```python
from build123d import *

# Parameters (mm, degrees)
F0_W     = 55.88
F0_H     = 105.1052
F0_R     = 1.7145
F0_W_2   = 48.26
F0_H_2   = 10.4902
F1_DEPTH = 3.175
F2_R     = 1.016
F3_DEPTH = 105.1062
F4_R     = 1.7145
F4_W     = 9.3726
F4_H     = 6.35
F4_W_2   = 6.223
F4_H_2   = 10.414
F4_W_3   = 8.3566
F4_H_3   = 15.24
F5_DEPTH = 3.175
F6_W     = 7.62
F6_H     = 10.16
F6_W_2   = 5.08
F6_H_2   = 6.35
F7_DEPTH = 25.4
F8_R     = 1.6002
F9_R     = 3.175
F10_F1_R = 1.016
F10_F2_R = 1.016


# Not quite as in the source:
# - a feature names something its author has since deleted; it is built from what else it names


with BuildPart() as f1:
    # F0 (on Top) → F1 (new body)
    with BuildSketch(Plane.XY):
        Rectangle(F0_W, F0_H)
        with Locations((-17.9451, -29.5656)):
            Circle(F0_R, mode=Mode.SUBTRACT)
        with Locations((-9.8679, -47.7901)):
            Circle(F0_R, mode=Mode.SUBTRACT)
        with Locations((9.8679, -47.7901)):
            Circle(F0_R, mode=Mode.SUBTRACT)
        with Locations((-9.8679, 15.0622)):
            Circle(F0_R, mode=Mode.SUBTRACT)
        with Locations((0, 37.7825)):
            Rectangle(F0_W_2, F0_H_2, mode=Mode.SUBTRACT)
        with Locations((-9.8679, 47.7901)):
            Circle(F0_R, mode=Mode.SUBTRACT)
        with Locations((9.8679, 15.0622)):
            Circle(F0_R, mode=Mode.SUBTRACT)
        with Locations((9.8679, 47.7901)):
            Circle(F0_R, mode=Mode.SUBTRACT)
    extrude(amount=F1_DEPTH)

    # F2 (on face) → F3 (cut, through all)
    with BuildSketch(Plane.XZ.offset(52.5526)):
        Circle(F2_R)
    extrude(amount=-F3_DEPTH, mode=Mode.SUBTRACT)

    # F4 (on face) → F5 (join)
    with BuildSketch(Plane.XY.offset(3.175)):
        Polygon((-7.3914, 17.7927), (-20.5994, 17.7927), (-20.5994, 14.8093839596), (-20.5994, 9.8679), (-14.7574, 9.8679), (-14.7574, 13.9827), (-11.8364, 13.9827), (-11.8364, 12.2047), (-7.3914, 12.2047), (-7.3914, 13.9827), align=None)
        with Locations((-9.8679, 15.0622)):
            Circle(F4_R, mode=Mode.SUBTRACT)
        with Locations((11.3157, 14.6177)):
            Rectangle(F4_W, F4_H)
        with Locations((9.8679, 15.0622)):
            Circle(F4_R, mode=Mode.SUBTRACT)
        with Locations((-17.4879, -28.6893)):
            Rectangle(F4_W_2, F4_H_2)
        with Locations((-17.9451, -29.5656)):
            Circle(F4_R, mode=Mode.SUBTRACT)
        with Locations((16.2687, -22.6695)):
            Rectangle(F4_W_3, F4_H_3)
    extrude(amount=F5_DEPTH)

    # F6 (on face) → F7 (cut)
    with BuildSketch(Plane(origin=(0, 0, 0), x_dir=(1, 0, 0), z_dir=(0, 0, -1))):
        with Locations((14.9225, 4.4323)):
            Rectangle(F6_W, F6_H)
        with Locations((-13.6525, 2.5273)):
            Rectangle(F6_W_2, F6_H_2)
    extrude(amount=-F7_DEPTH, mode=Mode.SUBTRACT)

    # F8
    f8_edges = [f1.edges().sort_by_distance(p)[0] for p in [
        (-16.1925, 0.6477, 1.5875),
        (11.1125, 0.6477, 1.5875),
        (18.7325, 0.6477, 1.5875),
        (18.7325, -9.5123, 1.5875),
        (11.1125, -9.5123, 1.5875),
        (-16.1925, -5.7023, 1.5875),
        (-11.1125, -5.7023, 1.5875),
        (-11.1125, 0.6477, 1.5875),
    ]]
    fillet(f8_edges, radius=F8_R)

    # F9
    f9_edges = [f1.edges().sort_by_distance(p)[0] for p in [
        (-24.13, 32.5374, 1.5875),
        (24.13, 32.5374, 1.5875),
        (24.13, 43.0276, 1.5875),
        (-24.13, 43.0276, 1.5875),
    ]]
    fillet(f9_edges, radius=F9_R)

    # F10: fillet of radius 1.016 on 34 edges, made by hand

    # F10_f1
    f10_f1_edges = [f1.edges().sort_by_distance(p)[0] for p in [
        (-7.3914, 17.7927, 4.7625),
        (6.6294, 17.7927, 4.7625),
        (16.002, 17.7927, 4.7625),
        (20.447, -15.0495, 4.7625),
        (12.0904, -15.0495, 4.7625),
        (20.447, -30.2895, 4.7625),
        (12.0904, -30.2895, 4.7625),
        (-14.3764, -33.8963, 4.7625),
        (-20.5994, -33.8963, 4.7625),
        (-14.3764, -23.4823, 4.7625),
        (-20.5994, -23.4823, 4.7625),
        (6.6294, 11.4427, 4.7625),
        (16.002, 11.4427, 4.7625),
        (-20.5994, 17.7927, 4.7625),
        (-20.5994, 9.8679, 4.7625),
        (-14.7574, 9.8679, 4.7625),
        (-7.3914, 12.2047, 4.7625),
        (-11.8364, 12.2047, 4.7625),
    ]]
    fillet(f10_f1_edges, radius=F10_F1_R)

    # F10_f2
    f10_f2_edges = [f1.edges().sort_by_distance(p)[0] for p in [
        (-14.3764, -28.6893, 3.175),
        (20.447, -22.6695, 3.175),
        (16.002, 14.6177, 3.175),
        (-7.3914, 14.9987, 3.175),
        (-20.5994, -28.6893, 3.175),
        (-17.4879, -23.4823, 3.175),
        (-17.4879, -33.8963, 3.175),
        (16.2687, -30.2895, 3.175),
        (16.2687, -15.0495, 3.175),
        (12.0904, -22.6695, 3.175),
        (-13.9954, 17.7927, 3.175),
        (-20.5994, 13.8303, 3.175),
        (-17.6784, 9.8679, 3.175),
        (11.3157, 11.4427, 3.175),
        (11.3157, 17.7927, 3.175),
        (6.6294, 14.6177, 3.175),
        (6.9269795103, 17.4951204897, 3.175),
        (6.9269795103, 11.7402795103, 3.175),
        (15.7044204897, 17.4951204897, 3.175),
        (15.7044204897, 11.7402795103, 3.175),
        (-20.3018204897, 10.1654795103, 3.175),
        (-15.0549795103, 10.1654795103, 3.175),
        (-20.3018204897, 17.4951204897, 3.175),
        (-7.6889795103, 17.4951204897, 3.175),
        (12.3879795103, -15.3470795103, 3.175),
        (12.3879795103, -29.9919204897, 3.175),
        (20.1494204897, -15.3470795103, 3.175),
        (20.1494204897, -29.9919204897, 3.175),
        (-20.3018204897, -33.5987204897, 3.175),
        (-14.6739795103, -33.5987204897, 3.175),
        (-14.6739795103, -23.7798795103, 3.175),
        (-20.3018204897, -23.7798795103, 3.175),
        (-7.6889795103, 12.5022795103, 3.175),
    ]]
    fillet(f10_f2_edges, radius=F10_F2_R)


solid = f1.part
```
Can you work these out from the model? Positions are in its coordinate system, mm. A direction names the side the tool comes from. Round coordinates to 2 decimals unless told otherwise and drop trailing zeros. Loops run counter-clockwise (first coordinate to the right, second up) from the corner with the lowest first, then second, coordinate; pieces in that order, holes last.
Item 1: Which directions (+Z, -Z, +X, -X, +Y, -Y) give clear straight access to the entire face, cutting with the end or side of a thin tool? Please do faces 1 (the flat face through (-7.391, 15, 5)), 2 (the flat face through (16.002, 15, 5)), 3 (the flat face through (-16.192, -3, 2)), 4 (the flat face through (11, 11.443, 5)).
Item 2: Please list where these lines run through material, in increasing order: L1, parallel to X at y = -1.5, z = 2.5; L2, parallel to Y at x = 17, z = 1; L3, parallel to Y at x = -16, z = 3.
Item 3: If we mould it in two halves opening along X, with no side actions, what happens to faces 5 (the flat face through (20.447, -23, 5)), 6 (the flat face through (-14, 0.648, 2)), 7 (the flat face through (-15, 1, 0))? For each: +X half, -X half, draft (parallel to the pull), parting line (faces both ways), or undercut.
Item 4: Suppose I cut it at A-A, the plane x = 4.5. Write out the boundary of the cut face in (y, z) (3 decimals), then the cut area to 3 significant figures.
Item 5: Will these pins go through, and if not, where does the flat tip stop? pin 1 Ø8 at (x, y) = (-14.5, -14) entering from +Z (3 decimals); pin 2 Ø0.6 at (y, z) = (-28, 5.5) entering from +X; pin 3 Ø1.7 at (x, z) = (15, 5) entering from +Y.
Item 6: Suppose I cut it at B-B, the plane y = -39. Write out the boundary of the cut face in (x, z) (3 decimals).
Reported:
1. face 1: +Z, +Y, -Y
1. face 2: +Z, +X, +Y
1. face 3: +Z, -Z
1. face 4: +Z, +X
2. L1: x = -27.94 to -16.19, -11.11 to 11.11, 18.73 to 27.94
2. L2: y = -52.55 to -9.51, 0.65 to 32.54, 43.03 to 52.55
2. L3: y = -52.55 to -4.86, -0.19 to 32.54, 43.03 to 52.55
3. face 5: +X half
3. face 6: undercut
3. face 7: draft
4. outline: (-52.553, 0) - (32.537, 0) - (32.537, 3.175) - (-52.553, 3.175) - close; (43.028, 0) - (52.553, 0) - (52.553, 3.175) - (43.028, 3.175) - close
4. area: 300 mm2
5. pin 1: stops at z = 3.175
5. pin 2: stops at x = 20.45
5. pin 3: stops at y = 17.79
6. outline: (-27.94, 0) - (-1.016, 0) arc R1.016 cw to (1.016, 0) - (27.94, 0) - (27.94, 3.175) - (-27.94, 3.175) - close
